Could you check a few things on this drawing? It's one solid part, dimensions in mm from its lowest x, y, z. Give positions to 0.01 mm unless a question says otherwise; leave off trailing zeros. Order: outer loops, then holes, each group sorted by start corner. A loop starts at its lowest first (then second) coordinate and runs counter-clockwise, first axis right, second up.
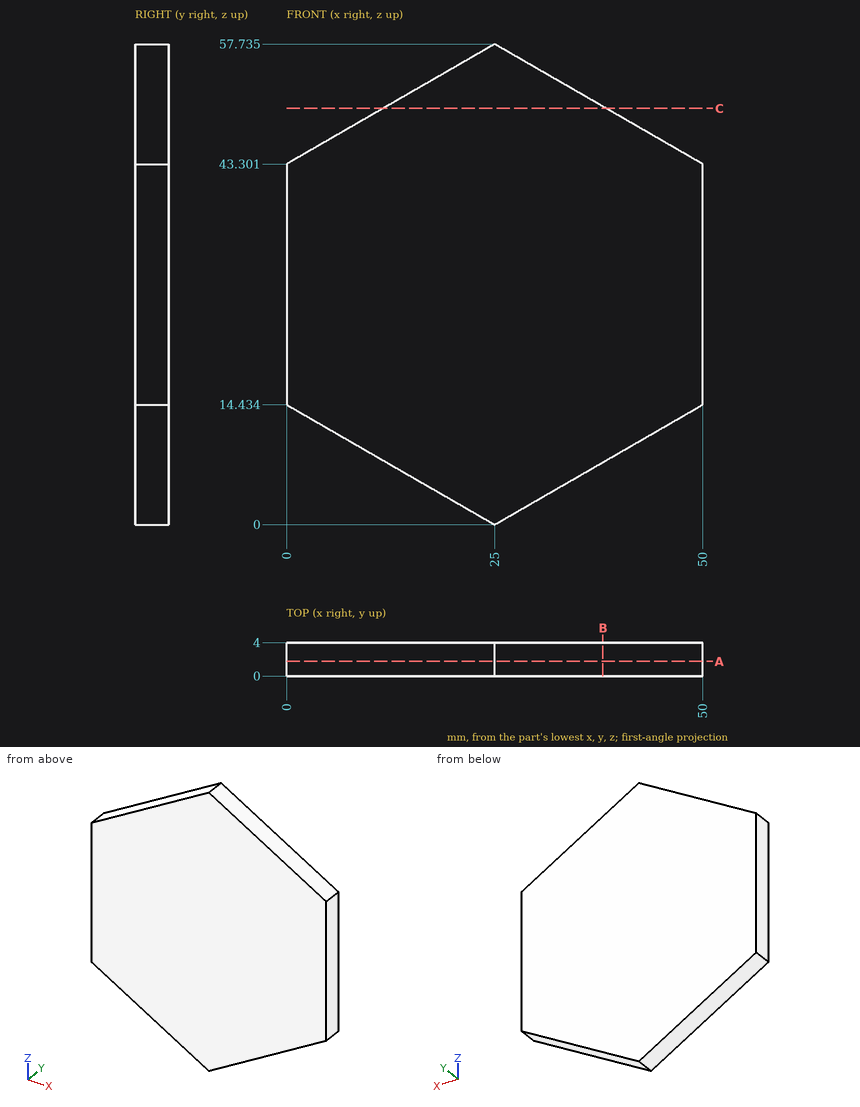
1) If I drill on line 1 (X direction, y = 3.65, z = 53.5) (1 decimal); line 2 (Z direction, x = 18, y = 3.05); line 3 (X direction, y = 1.2, z = 49), over which ranges is the centre line in solid material (lowest first)?
2) Suppose I cut it at C-C (z = 50). Please give me the cut outline in (x, y).
3) Suppose I cut it at A-A (y = 1.75). Please give me the cut outline in (x, z) (1 decimal).
4) I'm going to push a flat-ended pin straight in: pin 1 Ø1 at (x, y) = (20.5, 1) entering from +Z (1 decimal). Where does the tip first touch, or does it pass through?
5) Suppose I cut it at B-B (x = 38). Please give me the cut outline in (y, z) (1 decimal).
Results:
1. line 1: x = 17.7 to 32.3
1. line 2: z = 4.04 to 53.69
1. line 3: x = 9.87 to 40.13
2. outline: (11.6, 0) - (38.4, 0) - (38.4, 4) - (11.6, 4) - close
3. outline: (0, 14.4) - (25, 0) - (50, 14.4) - (50, 43.3) - (25, 57.7) - (0, 43.3) - close
4. pin 1: stops at z = 55.4
5. outline: (0, 7.5) - (4, 7.5) - (4, 50.2) - (0, 50.2) - close
